Can you work these out from the model? Positions are in its coordinate system, mm. A direction names the side the tool comes from. Coordinates: 2 decimals unless noted, no trailing zeros. Order: outer loops, then holes, each group sorted by start corner. A loop starts at its lowest first (then second) coordinate and runs counter-clockwise, first axis right, second up. Notation, with made-up numbers: (-25.75, 22.5) -> (-21.75, 22.5) arc R26 ccw to (-21.75, 51.5) -> close; hole circle Ø5 at (71.5, 75.5). An arc over 180 degrees is marked (long way). Answer in a Markdown table with one row per item.
```python
from build123d import *

# Parameters (mm, degrees)
F0_R     = 38
F0_R_2   = 7.5
F1_DEPTH = 1.5
F2_R     = 38
F2_R_2   = 36
F2_R_3   = 12.5
F2_R_4   = 10.5
F3_DEPTH = 15
F4_SIZE  = 0.75
F5_R     = 3
F6_DEPTH = 1.501


with BuildPart() as f1:
    # F0 (on Top) → F1 (new body)
    with BuildSketch(Plane.XY):
        Circle(F0_R)
        with Locations((-17.5, -17.5)):
            Circle(F0_R_2, mode=Mode.SUBTRACT)
        with Locations((17.5, -17.5)):
            Circle(F0_R_2, mode=Mode.SUBTRACT)
        with Locations((-17.5, 17.5)):
            Circle(F0_R_2, mode=Mode.SUBTRACT)
        Circle(F0_R_2, mode=Mode.SUBTRACT)
        with Locations((17.5, 17.5)):
            Circle(F0_R_2, mode=Mode.SUBTRACT)
    extrude(amount=F1_DEPTH)

    # F2 (on face) → F3 (join)
    with BuildSketch(Plane.XY.offset(1.5)):
        Circle(F2_R)
        Circle(F2_R_2, mode=Mode.SUBTRACT)
        Circle(F2_R_3)
        Circle(F2_R_4, mode=Mode.SUBTRACT)
    extrude(amount=F3_DEPTH)

    # F4
    f4_edges = [f1.edges().sort_by_distance(p)[0] for p in [
        (-38, 0, 0),
        (-38, 0, 16.5),
        (-36, 0, 16.5),
        (-12.5, 0, 16.5),
        (-10.5, 0, 16.5),
    ]]
    chamfer(f4_edges, length=F4_SIZE)

    # F5 (on face) → F6 (cut, through all)
    with BuildSketch(Plane.XY.offset(1.5)):
        with Locations((-27, 0)):
            Circle(F5_R)
        with Locations((0, -27)):
            Circle(F5_R)
        with Locations((27, 0)):
            Circle(F5_R)
        with Locations((0, 27)):
            Circle(F5_R)
    extrude(amount=-F6_DEPTH, mode=Mode.SUBTRACT)


solid = f1.part
```
(1) We'd pull the mould along Y, two halves only. Please class faces 1 (the cylindrical face through (-30, 0, 1)), 2 (the flat face through (-16.73, -32.94, 16.5)): +Y half, -Y half, draft (parallel to the pull), parting line (faces both ways), or undercut.
Response values:
| item | result |
|---|---|
| face 1 | undercut |
| face 2 | draft |
(2) Will these pins go through, and if not, where does the flat tip stop? pin 1 Ø1 at (x, z) = (-14, 9.5) entering from +Y; pin 2 Ø19.5 at (x, y) = (-17.5, -17.5) entering from +Z; pin 3 Ø1.5 at (x, z) = (3.5, 11) entering from +Y.
Response values:
| item | result |
|---|---|
| pin 1 | y = 35.52 |
| pin 2 | z = 1.5 |
| pin 3 | y = 37.9 |
(3) Suppose I cut it at B-B (y = 0). Count the separate pieces of the cut face and the enclosed holes in it, and give its area (3 significant figures).
Response values:
| item | result |
|---|---|
| separate pieces | 4 |
| enclosed holes | 0 |
| area | 191 mm2 |
(4) Suppose I cut it at A-A (z = 8). Please give me the cut outline in (x, y), and give its area (3 significant figures).
Response values:
| item | result |
|---|---|
| outline | circle Ø76 at (0, 0); circle Ø25 at (0, 0); hole circle Ø72 at (0, 0); hole circle Ø21 at (0, 0) |
| area | 609 mm2 |
(5) On a 3-axis mill with a long thin cutter (end or side, diameter ignored), from which of +Z, -Z, +X, -X, +Y, -Y can I reach the whole of each face in a straight line? I mean faces 3 (the flat face through (-1, -8, 0)), 4 (the flat face through (-1, -15, 1.5)). Say none if no direction works.
Response values:
| item | result |
|---|---|
| face 3 | -Z, +X, -X, +Y, -Y |
| face 4 | +Z |
(6) I need wall thicknesses on line 1 (Y direction, x = 0, z = 0.85); line 2 (Y direction, x = -23.5, z = 1.25); line 3 (Y direction, x = 5.5, z = 8.5). Which ranges of each line are inside material? Lowest first, please. Write a range as [from, to].
Response values:
| item | result |
|---|---|
| line 1 | [-38, -30], [-24, -7.5], [7.5, 24], [30, 38] |
| line 2 | [-29.86, -22], [-13, 13], [22, 29.86] |
| line 3 | [-37.6, -35.58], [-11.22, -8.94], [8.94, 11.22], [35.58, 37.6] |
